```python
from build123d import *

# Parameters (mm, degrees)
SKETCH_3_R                   = 46
SKETCH_3_R_2                 = 34.6
EXTRUDE_2_DEPTH              = 3
SKETCH_5_R                   = 36
SKETCH_5_R_2                 = 33.5
EXTRUDE_3_DEPTH              = 5.49
SKETCH_2_R                   = 46
SKETCH_2_R_2                 = 41.6
EXTRUDE_1_DEPTH              = 2.98
SKETCH_6_R                   = 36
SKETCH_6_R_2                 = 30
EXTRUDE_4_DEPTH              = 1.5
EXTRUDE_5_DEPTH              = 3
EXTRUDE_5_DEPTH_BACK         = 2.98
SKETCH_12_W                  = 1.25
SKETCH_12_H                  = 5.98
HOLE_WIZARD_M3_1_AT_2_COUNT  = 2
HOLE_WIZARD_M3_1_AT_2_PITCH  = 64.085879878
HOLE_WIZARD_M3_1_AT_3_COUNT  = 2
HOLE_WIZARD_M3_1_AT_3_PITCH  = 71.478511138
HOLE_WIZARD_M3_1_AT_4_COUNT  = 2
HOLE_WIZARD_M3_1_AT_4_PITCH  = 73.999999995
HOLE_WIZARD_M3_1_AT_5_COUNT  = 2
HOLE_WIZARD_M3_1_AT_5_PITCH  = 19.15260934
HOLE_WIZARD_M3_1_AT_6_COUNT  = 2
HOLE_WIZARD_M3_1_AT_6_PITCH  = 36.999999998
HOLE_WIZARD_M3_1_AT_7_COUNT  = 2
HOLE_WIZARD_M3_1_AT_7_PITCH  = 52.325901805
HOLE_WIZARD_M3_1_AT_8_COUNT  = 2
HOLE_WIZARD_M3_1_AT_8_PITCH  = 71.47851114
HOLE_WIZARD_M3_1_AT_9_COUNT  = 2
HOLE_WIZARD_M3_1_AT_9_PITCH  = 64.085879872
HOLE_WIZARD_M3_1_AT_10_COUNT = 2
HOLE_WIZARD_M3_1_AT_10_PITCH = 52.325901805
HOLE_WIZARD_M3_1_AT_11_COUNT = 2
HOLE_WIZARD_M3_1_AT_11_PITCH = 36.999999994
HOLE_WIZARD_M3_1_AT_12_COUNT = 2
HOLE_WIZARD_M3_1_AT_12_PITCH = 19.152609334
CUT_EXTRUDE_1_REACH          = 8.99
SKETCH_13_R                  = 1.25
SKETCH_13_R_2                = 2.2
SKETCH_25_R                  = 3.25
CUT_EXTRUDE_9_DEPTH          = 10
EXTRUDE_7_DEPTH              = 4
EXTRUDE_7_DEPTH_BACK         = 2
FILLET_1_R                   = 5
SKETCH_27_W                  = 100
SKETCH_27_H                  = 92
CUT_EXTRUDE_10_DEPTH         = 10.99
CUT_EXTRUDE_10_DEPTH_BACK    = 40.48


with BuildPart() as part:
    # 草图3 → 凸台-拉伸2 (new body)
    with BuildSketch(Plane.XY):
        Circle(SKETCH_3_R)
        Circle(SKETCH_3_R_2, mode=Mode.SUBTRACT)
    extrude(amount=EXTRUDE_2_DEPTH)

    # 草图5 → 凸台-拉伸3 (add)
    with BuildSketch(Plane.XY.offset(3)):
        Circle(SKETCH_5_R)
        Circle(SKETCH_5_R_2, mode=Mode.SUBTRACT)
    extrude(amount=EXTRUDE_3_DEPTH)

    # 草图2 → 凸台-拉伸1 (add)
    with BuildSketch(Plane.XY):
        Circle(SKETCH_2_R)
        Circle(SKETCH_2_R_2, mode=Mode.SUBTRACT)
    extrude(amount=-EXTRUDE_1_DEPTH)

    # 草图6 → 凸台-拉伸4 (add)
    with BuildSketch(Plane.XY.offset(8.49)):
        Circle(SKETCH_6_R)
        Circle(SKETCH_6_R_2, mode=Mode.SUBTRACT)
    extrude(amount=EXTRUDE_4_DEPTH)

    # 草图8 → 凸台-拉伸5 (add, two sides)
    with BuildSketch(Plane.XY) as extrude_5_sk:
        with BuildLine():
            Line((-50, 20.008021569), (-45.01389718, 20.008021569))
            ThreePointArc((-45.01389718, 20.008021569), (-42.026432396, 20.80859551), (-39.839615313, 22.995761603))
            ThreePointArc((-39.839615313, 22.995761603), (-46, 0), (-39.839615313, -22.995761603))
            ThreePointArc((-39.839615313, -22.995761603), (-42.026432396, -20.80859551), (-45.01389718, -20.008021569))
            Line((-45.01389718, -20.008021569), (-50, -20.008021569))
            Line((-50, -20.008021569), (-50, 20.008021569))
        make_face()
    extrude(amount=EXTRUDE_5_DEPTH)
    extrude(extrude_5_sk.sketch, amount=-EXTRUDE_5_DEPTH_BACK)

    # 草图12 → M3 螺纹孔的螺纹孔钻头1 (revolve, cut)
    with BuildSketch(Plane(origin=(-35.73925557, -9.57630467, 3), x_dir=(0, -1, 0), z_dir=(1, 0, 0))):
        with Locations((0.625, 2.99)):
            Rectangle(SKETCH_12_W, SKETCH_12_H)
    hole_wizard_m3_1 = revolve(axis=Axis((-35.73925557, -9.57630467, 9.35), (0, 0, -1)), mode=Mode.SUBTRACT)

    # M3 螺纹孔的螺纹孔钻头1 at 2: M3 螺纹孔的螺纹孔钻头1 ×2
    with Locations(*[Vector(0.707106781, 0.707106781, 0) * (i * HOLE_WIZARD_M3_1_AT_2_PITCH) for i in range(1, HOLE_WIZARD_M3_1_AT_2_COUNT)]):
        add(hole_wizard_m3_1, mode=Mode.SUBTRACT)

    # M3 螺纹孔的螺纹孔钻头1 at 3: M3 螺纹孔的螺纹孔钻头1 ×2
    with Locations(*[Vector(0.866025404, 0.5, 0) * (i * HOLE_WIZARD_M3_1_AT_3_PITCH) for i in range(1, HOLE_WIZARD_M3_1_AT_3_COUNT)]):
        add(hole_wizard_m3_1, mode=Mode.SUBTRACT)

    # M3 螺纹孔的螺纹孔钻头1 at 4: M3 螺纹孔的螺纹孔钻头1 ×2
    with Locations(*[Vector(0.965925826, 0.258819045, 0) * (i * HOLE_WIZARD_M3_1_AT_4_PITCH) for i in range(1, HOLE_WIZARD_M3_1_AT_4_COUNT)]):
        add(hole_wizard_m3_1, mode=Mode.SUBTRACT)

    # M3 螺纹孔的螺纹孔钻头1 at 5: M3 螺纹孔的螺纹孔钻头1 ×2
    with Locations(*[(0, i * HOLE_WIZARD_M3_1_AT_5_PITCH, 0) for i in range(1, HOLE_WIZARD_M3_1_AT_5_COUNT)]):
        add(hole_wizard_m3_1, mode=Mode.SUBTRACT)

    # M3 螺纹孔的螺纹孔钻头1 at 6: M3 螺纹孔的螺纹孔钻头1 ×2
    with Locations(*[Vector(0.258819045, 0.965925826, 0) * (i * HOLE_WIZARD_M3_1_AT_6_PITCH) for i in range(1, HOLE_WIZARD_M3_1_AT_6_COUNT)]):
        add(hole_wizard_m3_1, mode=Mode.SUBTRACT)

    # M3 螺纹孔的螺纹孔钻头1 at 7: M3 螺纹孔的螺纹孔钻头1 ×2
    with Locations(*[Vector(0.5, 0.866025404, 0) * (i * HOLE_WIZARD_M3_1_AT_7_PITCH) for i in range(1, HOLE_WIZARD_M3_1_AT_7_COUNT)]):
        add(hole_wizard_m3_1, mode=Mode.SUBTRACT)

    # M3 螺纹孔的螺纹孔钻头1 at 8: M3 螺纹孔的螺纹孔钻头1 ×2
    with Locations(*[(i * HOLE_WIZARD_M3_1_AT_8_PITCH, 0, 0) for i in range(1, HOLE_WIZARD_M3_1_AT_8_COUNT)]):
        add(hole_wizard_m3_1, mode=Mode.SUBTRACT)

    # M3 螺纹孔的螺纹孔钻头1 at 9: M3 螺纹孔的螺纹孔钻头1 ×2
    with Locations(*[Vector(0.965925826, -0.258819045, 0) * (i * HOLE_WIZARD_M3_1_AT_9_PITCH) for i in range(1, HOLE_WIZARD_M3_1_AT_9_COUNT)]):
        add(hole_wizard_m3_1, mode=Mode.SUBTRACT)

    # M3 螺纹孔的螺纹孔钻头1 at 10: M3 螺纹孔的螺纹孔钻头1 ×2
    with Locations(*[Vector(0.866025404, -0.5, 0) * (i * HOLE_WIZARD_M3_1_AT_10_PITCH) for i in range(1, HOLE_WIZARD_M3_1_AT_10_COUNT)]):
        add(hole_wizard_m3_1, mode=Mode.SUBTRACT)

    # M3 螺纹孔的螺纹孔钻头1 at 11: M3 螺纹孔的螺纹孔钻头1 ×2
    with Locations(*[Vector(0.707106781, -0.707106781, 0) * (i * HOLE_WIZARD_M3_1_AT_11_PITCH) for i in range(1, HOLE_WIZARD_M3_1_AT_11_COUNT)]):
        add(hole_wizard_m3_1, mode=Mode.SUBTRACT)

    # M3 螺纹孔的螺纹孔钻头1 at 12: M3 螺纹孔的螺纹孔钻头1 ×2
    with Locations(*[Vector(0.5, -0.866025404, 0) * (i * HOLE_WIZARD_M3_1_AT_12_PITCH) for i in range(1, HOLE_WIZARD_M3_1_AT_12_COUNT)]):
        add(hole_wizard_m3_1, mode=Mode.SUBTRACT)

    # 草图13 → 切除-拉伸1 (cut, up to next)
    with BuildSketch(Plane.XY.offset(3), mode=Mode.PRIVATE) as cut_extrude_1_sk1:
        with Locations((-35.73925557, -9.57630467)):
            Circle(SKETCH_13_R)
    cut_extrude_1_tool1 = extrude(cut_extrude_1_sk1.sketch, amount=CUT_EXTRUDE_1_REACH, mode=Mode.PRIVATE) & part.part
    add(cut_extrude_1_tool1.solids().sort_by_distance((-35.739256, -9.576305, 3))[0], mode=Mode.SUBTRACT)
    # 草图13 → 切除-拉伸1 (cut, up to next)
    with BuildSketch(Plane.XY.offset(3), mode=Mode.PRIVATE) as cut_extrude_1_sk2:
        with Locations((-26.1629509, -26.1629509)):
            Circle(SKETCH_13_R_2)
    cut_extrude_1_tool2 = extrude(cut_extrude_1_sk2.sketch, amount=CUT_EXTRUDE_1_REACH, mode=Mode.PRIVATE) & part.part
    add(cut_extrude_1_tool2.solids().sort_by_distance((-26.162951, -26.162951, 3))[0], mode=Mode.SUBTRACT)
    # 草图13 → 切除-拉伸1 (cut, up to next)
    with BuildSketch(Plane.XY.offset(3), mode=Mode.PRIVATE) as cut_extrude_1_sk3:
        with Locations((-35.73925557, 9.57630467)):
            Circle(SKETCH_13_R)
    cut_extrude_1_tool3 = extrude(cut_extrude_1_sk3.sketch, amount=CUT_EXTRUDE_1_REACH, mode=Mode.PRIVATE) & part.part
    add(cut_extrude_1_tool3.solids().sort_by_distance((-35.739256, 9.576305, 3))[0], mode=Mode.SUBTRACT)
    # 草图13 → 切除-拉伸1 (cut, up to next)
    with BuildSketch(Plane.XY.offset(3), mode=Mode.PRIVATE) as cut_extrude_1_sk4:
        with Locations((-26.1629509, 26.1629509)):
            Circle(SKETCH_13_R_2)
    cut_extrude_1_tool4 = extrude(cut_extrude_1_sk4.sketch, amount=CUT_EXTRUDE_1_REACH, mode=Mode.PRIVATE) & part.part
    add(cut_extrude_1_tool4.solids().sort_by_distance((-26.162951, 26.162951, 3))[0], mode=Mode.SUBTRACT)
    # 草图13 → 切除-拉伸1 (cut, up to next)
    with BuildSketch(Plane.XY.offset(3), mode=Mode.PRIVATE) as cut_extrude_1_sk5:
        with Locations((-9.57630467, 35.73925557)):
            Circle(SKETCH_13_R_2)
    cut_extrude_1_tool5 = extrude(cut_extrude_1_sk5.sketch, amount=CUT_EXTRUDE_1_REACH, mode=Mode.PRIVATE) & part.part
    add(cut_extrude_1_tool5.solids().sort_by_distance((-9.576305, 35.739256, 3))[0], mode=Mode.SUBTRACT)
    # 草图13 → 切除-拉伸1 (cut, up to next)
    with BuildSketch(Plane.XY.offset(3), mode=Mode.PRIVATE) as cut_extrude_1_sk6:
        with Locations((26.1629509, 26.1629509)):
            Circle(SKETCH_13_R_2)
    cut_extrude_1_tool6 = extrude(cut_extrude_1_sk6.sketch, amount=CUT_EXTRUDE_1_REACH, mode=Mode.PRIVATE) & part.part
    add(cut_extrude_1_tool6.solids().sort_by_distance((26.162951, 26.162951, 3))[0], mode=Mode.SUBTRACT)
    # 草图13 → 切除-拉伸1 (cut, up to next)
    with BuildSketch(Plane.XY.offset(3), mode=Mode.PRIVATE) as cut_extrude_1_sk7:
        with Locations((35.73925557, 9.57630467)):
            Circle(SKETCH_13_R)
    cut_extrude_1_tool7 = extrude(cut_extrude_1_sk7.sketch, amount=CUT_EXTRUDE_1_REACH, mode=Mode.PRIVATE) & part.part
    add(cut_extrude_1_tool7.solids().sort_by_distance((35.739256, 9.576305, 3))[0], mode=Mode.SUBTRACT)
    # 草图13 → 切除-拉伸1 (cut, up to next)
    with BuildSketch(Plane.XY.offset(3), mode=Mode.PRIVATE) as cut_extrude_1_sk8:
        with Locations((35.73925557, -9.57630467)):
            Circle(SKETCH_13_R)
    cut_extrude_1_tool8 = extrude(cut_extrude_1_sk8.sketch, amount=CUT_EXTRUDE_1_REACH, mode=Mode.PRIVATE) & part.part
    add(cut_extrude_1_tool8.solids().sort_by_distance((35.739256, -9.576305, 3))[0], mode=Mode.SUBTRACT)
    # 草图13 → 切除-拉伸1 (cut, up to next)
    with BuildSketch(Plane.XY.offset(3), mode=Mode.PRIVATE) as cut_extrude_1_sk9:
        with Locations((9.57630467, -35.73925557)):
            Circle(SKETCH_13_R_2)
    cut_extrude_1_tool9 = extrude(cut_extrude_1_sk9.sketch, amount=CUT_EXTRUDE_1_REACH, mode=Mode.PRIVATE) & part.part
    add(cut_extrude_1_tool9.solids().sort_by_distance((9.576305, -35.739256, 3))[0], mode=Mode.SUBTRACT)
    # 草图13 → 切除-拉伸1 (cut, up to next)
    with BuildSketch(Plane.XY.offset(3), mode=Mode.PRIVATE) as cut_extrude_1_sk10:
        with Locations((-9.57630467, -35.73925557)):
            Circle(SKETCH_13_R_2)
    cut_extrude_1_tool10 = extrude(cut_extrude_1_sk10.sketch, amount=CUT_EXTRUDE_1_REACH, mode=Mode.PRIVATE) & part.part
    add(cut_extrude_1_tool10.solids().sort_by_distance((-9.576305, -35.739256, 3))[0], mode=Mode.SUBTRACT)
    # 草图13 → 切除-拉伸1 (cut, up to next)
    with BuildSketch(Plane.XY.offset(3), mode=Mode.PRIVATE) as cut_extrude_1_sk11:
        with Locations((9.57630467, 35.73925557)):
            Circle(SKETCH_13_R_2)
    cut_extrude_1_tool11 = extrude(cut_extrude_1_sk11.sketch, amount=CUT_EXTRUDE_1_REACH, mode=Mode.PRIVATE) & part.part
    add(cut_extrude_1_tool11.solids().sort_by_distance((9.576305, 35.739256, 3))[0], mode=Mode.SUBTRACT)
    # 草图13 → 切除-拉伸1 (cut, up to next)
    with BuildSketch(Plane.XY.offset(3), mode=Mode.PRIVATE) as cut_extrude_1_sk12:
        with Locations((26.1629509, -26.1629509)):
            Circle(SKETCH_13_R_2)
    cut_extrude_1_tool12 = extrude(cut_extrude_1_sk12.sketch, amount=CUT_EXTRUDE_1_REACH, mode=Mode.PRIVATE) & part.part
    add(cut_extrude_1_tool12.solids().sort_by_distance((26.162951, -26.162951, 3))[0], mode=Mode.SUBTRACT)

    # 草图25 → 切除-拉伸9 (cut)
    with BuildSketch(Plane.XY.offset(3)):
        with Locations((-9.57630467, 35.73925557)):
            Circle(SKETCH_25_R)
        with Locations((-26.1629509, 26.1629509)):
            Circle(SKETCH_25_R)
        with Locations((-35.73925557, 9.57630467)):
            Circle(SKETCH_25_R)
        with Locations((-35.73925557, -9.57630467)):
            Circle(SKETCH_25_R)
        with Locations((-26.1629509, -26.1629509)):
            Circle(SKETCH_25_R)
        with Locations((-9.57630467, -35.73925557)):
            Circle(SKETCH_25_R)
    extrude(amount=CUT_EXTRUDE_9_DEPTH, mode=Mode.SUBTRACT)

    # 草图26 → 凸台-拉伸7 (add, two sides)
    with BuildSketch(Plane.ZY.offset(50)) as extrude_7_sk:
        with BuildLine():
            ThreePointArc((-12.98, 26.5), (-39.48, 0), (-12.98, -26.5))
            ThreePointArc((-12.98, -26.5), (-9.999377331, -25.617338519), (-7.98, -23.254010785))
            ThreePointArc((-7.98, -23.254010785), (-5.960622669, -20.89068305), (-2.98, -20.008021569))
            Line((-2.98, -20.008021569), (3, -20.008021569))
            Line((3, -20.008021569), (3, 20.008021569))
            Line((3, 20.008021569), (-2.98, 20.008021569))
            ThreePointArc((-2.98, 20.008021569), (-5.960622669, 20.89068305), (-7.98, 23.254010785))
            ThreePointArc((-7.98, 23.254010785), (-9.999377331, 25.617338519), (-12.98, 26.5))
        make_face()
    extrude(amount=EXTRUDE_7_DEPTH)
    extrude(extrude_7_sk.sketch, amount=-EXTRUDE_7_DEPTH_BACK)

    # 圆角1
    fillet_1_edges = [part.edges().sort_by_distance(p)[0] for p in [
        (-54, 0, 3),
    ]]
    fillet(fillet_1_edges, radius=FILLET_1_R)

    # 草图27 → 切除-拉伸10 (cut, two sides)
    with BuildSketch(Plane.XY) as cut_extrude_10_sk:
        with Locations((-50, 0)):
            Rectangle(SKETCH_27_W, SKETCH_27_H)
    extrude(amount=CUT_EXTRUDE_10_DEPTH, mode=Mode.SUBTRACT)
    extrude(cut_extrude_10_sk.sketch, amount=-CUT_EXTRUDE_10_DEPTH_BACK, mode=Mode.SUBTRACT)


solid = part.part
```
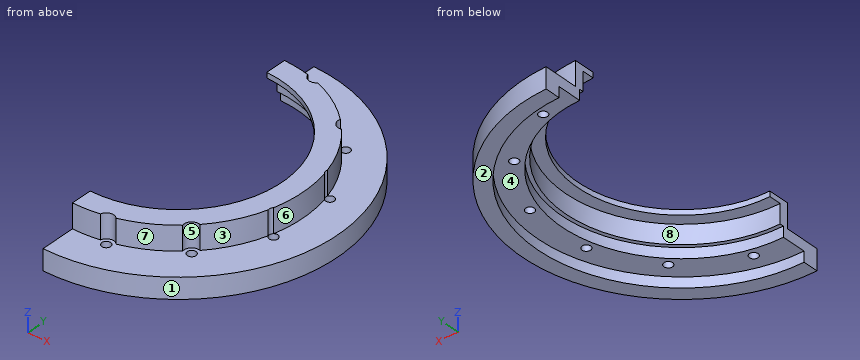
Part model, mm, in its own coordinate system. Face numbers are marked on the shaded views. A direction names the side the tool comes from. Give positions to 0.01 mm unless a question says otherwise; leave off trailing zeros. Write each loop counter-clockwise with the first axis right and the second up, starting at its lowest first coordinate (ties: lowest second). Pieces come first, ordered by that corner, then holes. Notation, with made-up numbers: (55, -11) -> (80, -11) arc R24 cw to (80, 24) -> close; hole circle Ø8 at (-13, -2.5). An arc over 180 degrees is marked (long way). Put each result on its own line as item: value. Start each with the question number.
Item 1: Which spindle directions (+Z, -Z, +X, -X, +Y, -Y) get a long thin tool onto all of the face, cutting with end or side? Do the marked faces 5, 6, 7 and 8. Say none if no direction does.
Item 2: Wall check: L1, parallel to Z at x = 39, y = -15; L2, parallel to Y at x = 10, z = 0.25; L3, parallel to Z at x = 28.5, y = -16. Give the ranges that are in metal, low to high. Write a range as [from, to].
Item 3: Cut at D-D (x = 23). List the corners of the cut face in (y, z).
Item 4: Pull direction Y, two halves, no side cores. Call the marked faces 1, 2, 3 and 4: pulls with the +Y half, pulls with the -Y half, needs draft (parallel to the pull), parting line crosses it, or undercut.
Item 5: Pin check, flat tips, straight feed: pin 1 Ø3 at (x, y) = (35.74, -9.58) entering from -Z; pin 2 Ø21 at (x, y) = (14, -16) entering from -Z; pin 3 Ø4 at (x, y) = (9.58, -35.74) entering from +Z. Stop position of each tip, or through.
Item 6: Cut at A-A (x = 14.5). List the corners of the cut face in (y, z), then the cut area to 3 significant figures.
Item 7: Cut at B-B (y = 0). List the corners of the cut face in (x, z), then the cut area to 3 significant figures.
Item 8: Cut at C-C (z = 4.75). List the corners of the cut face in (x, y).
Answer list:
1. face 5: +Z
1. face 6: +Z, +X
1. face 7: +Z, +X, -Y
1. face 8: -Z, -X
2. L1: z = [-2.98, 3]
2. L2: y = [-44.9, -36.92], [-34.56, -33.12], [33.12, 34.56], [36.92, 44.9]
2. L3: z = [8.49, 9.99]
3. outline: (-39.84, -2.98) -> (-34.66, -2.98) -> (-34.66, 0) -> (-25.85, 0) -> (-25.85, 3) -> (-24.36, 3) -> (-24.36, 8.49) -> (-19.26, 8.49) -> (-19.26, 9.99) -> (-27.69, 9.99) -> (-27.69, 3) -> (-39.84, 3) -> close; (19.26, 8.49) -> (24.36, 8.49) -> (24.36, 3) -> (25.85, 3) -> (25.85, 0) -> (34.66, 0) -> (34.66, -2.98) -> (39.84, -2.98) -> (39.84, 3) -> (27.69, 3) -> (27.69, 9.99) -> (19.26, 9.99) -> close
4. face 1: parting line crosses it
4. face 2: needs draft
4. face 3: pulls with the -Y half
4. face 4: undercut
5. pin 1: stops at z = 0
5. pin 2: stops at z = 8.49
5. pin 3: stops at z = 3
6. outline: (-43.65, -2.98) -> (-38.99, -2.98) -> (-38.99, 0) -> (-31.42, 0) -> (-31.42, 3) -> (-30.2, 3) -> (-30.2, 8.49) -> (-26.26, 8.49) -> (-26.26, 9.99) -> (-32.95, 9.99) -> (-32.95, 3) -> (-43.65, 3) -> close; (26.26, 8.49) -> (30.2, 8.49) -> (30.2, 3) -> (31.42, 3) -> (31.42, 0) -> (38.99, 0) -> (38.99, -2.98) -> (43.65, -2.98) -> (43.65, 3) -> (32.95, 3) -> (32.95, 9.99) -> (26.26, 9.99) -> close
6. area: 152 mm2
7. outline: (30, 8.49) -> (33.5, 8.49) -> (33.5, 3) -> (34.6, 3) -> (34.6, 0) -> (41.6, 0) -> (41.6, -2.98) -> (46, -2.98) -> (46, 3) -> (36, 3) -> (36, 9.99) -> (30, 9.99) -> close
7. area: 70.0 mm2
8. outline: (0, -36) arc R36 ccw to (7.44, -35.22) arc R2.2 cw to (11.17, -34.22) arc R36 ccw to (24.05, -26.79) arc R2.2 cw to (26.79, -24.05) arc R36 ccw to (34.57, -10.03) arc R1.25 cw to (34.96, -8.6) arc R36 ccw to (34.96, 8.6) arc R1.25 cw to (34.57, 10.03) arc R36 ccw to (26.79, 24.05) arc R2.2 cw to (24.05, 26.79) arc R36 ccw to (11.17, 34.22) arc R2.2 cw to (7.44, 35.22) arc R36 ccw to (0, 36) -> (0, 33.5) arc R33.5 cw to (0, -33.5) -> close
